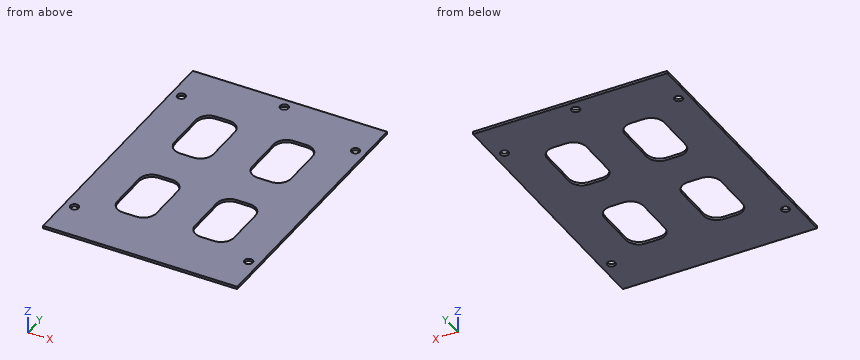
Autodesk Inventor part; units mm, degrees
ref_plane "YZ Plane" through (0, 0, 0) normal (1, 0, 0) x (0, 1, 0)
ref_plane "XZ Plane" through (0, 0, 0) normal (0, 1, 0) x (-1, 0, 0)
ref_plane "XY Plane" through (0, 0, 0) normal (0, 0, 1) x (1, 0, 0)
sketch "Sketch1" plane through (0, 0, 0) normal (0, 0, 1) x (1, 0, 0)
  line L0 (-37.5, 52.5) -> (37.5, 52.5)
  line L1 (37.5, 52.5) -> (37.5, -52.5)
  line L2 (37.5, -52.5) -> (-37.5, -52.5)
  line L3 (-37.5, -52.5) -> (-37.5, 52.5)
  line L4 (-37.5, 52.5) -> (37.5, -52.5) construction
  line L5 (37.5, 52.5) -> (-37.5, -52.5) construction
  circle A0 centre (33.6, -37.5) radius 1.6
  line L6 (0, 0) -> (12.8976, 0)
  line L7 (0, 0) -> (0, 11.3109)
  circle A1 centre (-33.6, -37.5) radius 1.6
  circle A2 centre (33.6, 37.5) radius 1.6
  circle A3 centre (-33.6, 37.5) radius 1.6
  circle A4 centre (0, 48.6) radius 1.6
  dimension "d0" = 75
  dimension "d1" = 105
  dimension "d2" = 3.2
  dimension "d3" = 3.9
  dimension "d4" = 15
  dimension "d11" = 3.2
  dimension "d12" = 3.9
extrude "Plate1" add sketch "Sketch1" along normal blind 1
sketch "Sketch2" plane through (0, 0, 1) normal (0, 0, 1) x (1, 0, 0)
  line L0 (-17.5, 32.5) -> (-12.5, 32.5)
  line L1 (-7.5, 27.5) -> (-7.5, 12.5)
  line L2 (-12.5, 7.5) -> (-17.5, 7.5)
  line L3 (-22.5, 12.5) -> (-22.5, 27.5)
  line L4 (-22.5, 32.5) -> (-7.5, 7.5) construction
  line L5 (-7.5, 32.5) -> (-22.5, 7.5) construction
  line L6 (0, 16.0345) -> (0, -16.0345)
  line L7 (-10.8621, 0) -> (10.8621, 0)
  arc A0 (-17.5, 32.5) -> (-22.5, 27.5) centre (-17.5, 27.5) ccw
  arc A1 (-7.5, 27.5) -> (-12.5, 32.5) centre (-12.5, 27.5) ccw
  arc A2 (-12.5, 7.5) -> (-7.5, 12.5) centre (-12.5, 12.5) ccw
  arc A3 (-22.5, 12.5) -> (-17.5, 7.5) centre (-17.5, 12.5) ccw
  line L8 (17.5, 32.5) -> (12.5, 32.5)
  line L9 (7.5, 27.5) -> (7.5, 12.5)
  line L10 (12.5, 7.5) -> (17.5, 7.5)
  line L11 (22.5, 12.5) -> (22.5, 27.5)
  line L12 (22.5, 32.5) -> (7.5, 7.5) construction
  line L13 (7.5, 32.5) -> (22.5, 7.5) construction
  arc A4 (22.5, 27.5) -> (17.5, 32.5) centre (17.5, 27.5) ccw
  arc A5 (12.5, 32.5) -> (7.5, 27.5) centre (12.5, 27.5) ccw
  arc A6 (7.5, 12.5) -> (12.5, 7.5) centre (12.5, 12.5) ccw
  arc A7 (17.5, 7.5) -> (22.5, 12.5) centre (17.5, 12.5) ccw
  line L14 (-17.5, -32.5) -> (-12.5, -32.5)
  line L15 (-7.5, -27.5) -> (-7.5, -12.5)
  line L16 (-12.5, -7.5) -> (-17.5, -7.5)
  line L17 (-22.5, -12.5) -> (-22.5, -27.5)
  line L18 (-22.5, -32.5) -> (-7.5, -7.5) construction
  line L19 (-7.5, -32.5) -> (-22.5, -7.5) construction
  arc A8 (-22.5, -27.5) -> (-17.5, -32.5) centre (-17.5, -27.5) ccw
  arc A9 (-12.5, -32.5) -> (-7.5, -27.5) centre (-12.5, -27.5) ccw
  arc A10 (-7.5, -12.5) -> (-12.5, -7.5) centre (-12.5, -12.5) ccw
  arc A11 (-17.5, -7.5) -> (-22.5, -12.5) centre (-17.5, -12.5) ccw
  arc A12 (12.5, -7.5) -> (7.5, -12.5) centre (12.5, -12.5) ccw
  line L20 (12.5, -7.5) -> (17.5, -7.5)
  arc A13 (22.5, -12.5) -> (17.5, -7.5) centre (17.5, -12.5) ccw
  line L21 (7.5, -27.5) -> (7.5, -12.5)
  line L22 (22.5, -12.5) -> (22.5, -27.5)
  arc A14 (7.5, -27.5) -> (12.5, -32.5) centre (12.5, -27.5) ccw
  line L23 (7.5, -32.5) -> (22.5, -7.5) construction
  line L24 (22.5, -32.5) -> (7.5, -7.5) construction
  line L25 (17.5, -32.5) -> (12.5, -32.5)
  arc A15 (17.5, -32.5) -> (22.5, -27.5) centre (17.5, -27.5) ccw
  point P0 (0, 0)
  point P1 (-15, 20)
  point P2 (0, 0)
  point P3 (15, 20)
  point P4 (-15, -20)
  point P5 (15, -20)
  dimension "d13" = 15
  dimension "d14" = 15
  dimension "d15" = 15
  dimension "d16" = 25
  dimension "d17" = 5
extrude "Cut1" cut sketch "Sketch2" against normal blind 1
equation "\"d18\" = 厚度"
equation "\"d5\" = 厚度"
equation "\"折彎半徑\" = 厚度"
equation "\"折彎離隙寬度\" = 厚度"
equation "\"折彎離隙深度\" = 0.5 * 厚度"
equation "\"轉角離隙大小\" = 4 * 厚度"
equation "\"最小剩餘\" = 2 * 厚度"
equation "\"轉移半徑\" = 折彎半徑"
equation "\"Jacobi半徑大小\" = 折彎半徑"
equation "\"間隙大小\" = 厚度"
properties part number "battery_box_24V_back" material "Aluminum"
CAD build for the part. Positions are in the model's coordinates, mm. Round coordinates to 2 decimals unless told otherwise and drop trailing zeros. Order: outer loops, then holes, each group sorted by start corner. A loop starts at its lowest first (then second) coordinate and runs counter-clockwise, first axis right, second up.
Q1. Drop a flat-ended pin along its axis: pin 1 (1.9 mm diameter, centred on x = 33.6, y = 37.5, fed in from -Z). Give the stop position or say it passes through.
Q2. Slice it at B-B (y = 48.6). Write the cut outline in (x, z).
Q3. Slice it at D-D (x = 0). Write the cut outline in (y, z).
Q4. Wall check: L1, parallel to X at y = 19, z = 0.25; L2, parallel to Y at x = 13.5, z = 0.75; L3, parallel to Y at x = -33.6, z = 0.7. Give the ranges that are in metal, low to high.
Q5. Slice it at A-A (y = -24). Write the cut outline in (x, z), and give its area (3 significant figures).
Q6. Slice it at C-C (x = 33.6). Write the cut outline in (y, z), and give its area (3 significant figures).
Results below:
1. pin 1: passes through
2. outline: (-37.5, 0) - (-1.6, 0) - (-1.6, 1) - (-37.5, 1) - close; (1.6, 0) - (37.5, 0) - (37.5, 1) - (1.6, 1) - close
3. outline: (-52.5, 0) - (47, 0) - (47, 1) - (-52.5, 1) - close; (50.2, 0) - (52.5, 0) - (52.5, 1) - (50.2, 1) - close
4. L1: x = -37.5 to -22.5, -7.5 to 7.5, 22.5 to 37.5
4. L2: y = -52.5 to -32.5, -7.5 to 7.5, 32.5 to 52.5
4. L3: y = -52.5 to -39.1, -35.9 to 35.9, 39.1 to 52.5
5. outline: (-37.5, 0) - (-22.5, 0) - (-22.5, 1) - (-37.5, 1) - close; (-7.5, 0) - (7.5, 0) - (7.5, 1) - (-7.5, 1) - close; (22.5, 0) - (37.5, 0) - (37.5, 1) - (22.5, 1) - close
5. area: 45.0 mm2
6. outline: (-52.5, 0) - (-39.1, 0) - (-39.1, 1) - (-52.5, 1) - close; (-35.9, 0) - (35.9, 0) - (35.9, 1) - (-35.9, 1) - close; (39.1, 0) - (52.5, 0) - (52.5, 1) - (39.1, 1) - close
6. area: 98.6 mm2
